Verification items for the finished model (mm, model axes). A direction names the side the tool comes from. Give positions to 0.01 mm unless a question says otherwise; leave off trailing zeros. Write each loop counter-clockwise with the first axis right and the second up, starting at its lowest first coordinate (ties: lowest second). Pieces come first, ordered by that corner, then holes. Notation, with made-up numbers: (80.5, 39) -> (92.5, 39) arc R20 ccw to (92.5, 49) -> close; hole circle Ø3 at (58, 72). An arc over 180 degrees is marked (long way). Write item = value, one per line.
from build123d import *

# Parameters (mm, degrees)
F0_W     = 7.5
F0_H     = 7.5
F1_DEPTH = 16.9418
F2_DEPTH = 12.7
F0_R     = 1.905
F3_DEPTH = 1.27


with BuildPart() as f1:
    # F0 (on Front) → F1 (new body)
    with BuildSketch(Plane.XZ):
        with BuildLine():
            ThreePointArc((7.504635, -5.86567), (9.005756, -3.101933), (9.525, 0))
            ThreePointArc((9.525, 0), (-3.140707, 8.992307), (-7.45381, -5.930121))
            ThreePointArc((-7.45381, -5.930121), (0.04104, -9.524912), (7.504635, -5.86567))
        make_face()
        Rectangle(F0_W, F0_H, mode=Mode.SUBTRACT)
    extrude(amount=-F1_DEPTH)

    # F0 (on Front) → F2 (join)
    with BuildSketch(Plane.XZ):
        with BuildLine():
            ThreePointArc((7.504635, -5.86567), (0.04104, -9.524912), (-7.45381, -5.930121))
            Line((-7.45381, -5.930121), (-7.45381, -63.01567))
            ThreePointArc((-7.45381, -63.01567), (0.025412, -70.494892), (7.504635, -63.01567))
            Line((7.504635, -63.01567), (7.504635, -5.86567))
        make_face()
    extrude(amount=-F2_DEPTH)

    # F0 (on Front) → F3 (join)
    with BuildSketch(Plane.XZ):
        Rectangle(F0_W, F0_H)
        Circle(F0_R, mode=Mode.SUBTRACT)
    extrude(amount=-F3_DEPTH)


solid = f1.part
Item 1: Go/stop test with flat-tipped pins: P1, Ø6.5, axis at y = 4, z = -38.5, coming from the -X side; P2, Ø4.5, axis at x = 0, z = 0, coming from the +Y side; P3, Ø1, axis at y = 7, z = -40, coming from the +X side. Record where each tip stops, or that it passes through.
Response values:
P1 = -7.45
P2 = 1.27
P3 = 7.5
Item 2: Sectioned sample at C-C on z = -39. Record the cut outline in (x, y), then the cut area to 3 significant figures.
Response values:
outline = (-7.45, 0) -> (7.5, 0) -> (7.5, 12.7) -> (-7.45, 12.7) -> close
area = 190 mm^2
Item 3: Sectioned sample at A-A on y = 14.5. Record the cut outline in (x, z) (3 decimals).
Response values:
outline = (-7.454, -5.93) arc R9.525 ccw to (9.525, 0) arc R9.525 ccw (long way) to start; hole (-3.75, -3.75) -> (3.75, -3.75) -> (3.75, 3.75) -> (-3.75, 3.75) -> close
Item 4: Material ranges on line 1 (Z direction, x = 0, y = 1) (3 decimals); line 2 (X direction, y = 6, z = -33); line 3 (Y direction, x = -6.5, z = -60), recorded low to high.
Response values:
line_1 = -70.495 to -1.905, 1.905 to 9.525
line_2 = -7.45 to 7.5
line_3 = 0 to 12.7
Item 5: Set-up check for faces 5 (the flat face through (3.75, 9, 0)), 6 (the flat face through (-7.454, 6, -34)), 7 (the cylindrical face through (-0.41, 0.63, -1.86)): record each of +Z, -Z, +X, -X, +Y, -Y from which the full face is reachable in a straight line by a thin tool's end or side.
Response values:
face_5 = +Y
face_6 = -Z, -X, +Y, -Y
face_7 = +Y, -Y
Item 6: Sectioned sample at D-D on y = 6.25. Record the cut outline in (x, z) (3 decimals).
Response values:
outline = (-7.454, -63.016) arc R7.479 ccw to (7.505, -63.016) -> (7.505, -5.866) arc R9.525 ccw to (9.525, 0) arc R9.525 ccw (long way) to (-7.454, -5.93) -> close; hole (-3.75, -3.75) -> (3.75, -3.75) -> (3.75, 3.75) -> (-3.75, 3.75) -> close
Item 7: Sectioned sample at B-B on x = 0. Record the cut outline in (y, z) (3 decimals).
Response values:
outline = (0, -70.495) -> (12.7, -70.495) -> (12.7, -9.525) -> (16.942, -9.525) -> (16.942, -3.75) -> (1.27, -3.75) -> (1.27, -1.905) -> (0, -1.905) -> close; (0, 1.905) -> (1.27, 1.905) -> (1.27, 3.75) -> (16.942, 3.75) -> (16.942, 9.525) -> (0, 9.525) -> close
Item 8: Mould release check, pull along Z, two halves, no side actions. Record for faces 1 (the cylindrical face through (-0.139, 6.261, -70.493)), 2 (the flat face through (0, 9, -3.75)), 3 (the flat face through (7.505, 6, -35)), 4 (the flat face through (0, 9, 3.75)): +Z half, -Z half, draft (parallel to the pull), parting line (faces both ways), or undercut.
Response values:
face_1 = -Z half
face_2 = undercut
face_3 = draft
face_4 = undercut
